from build123d import *

# Parameters (mm, degrees)
EXTRUDE_1_DEPTH     = 19
SKETCH_3_W          = 1
SKETCH_3_H          = 19
CUT_EXTRUDE_1_DEPTH = 1
SKETCH_4_R          = 2.25
CUT_EXTRUDE_2_DEPTH = 2
SKETCH_5_R          = 2.25
CUT_EXTRUDE_3_DEPTH = 2


with BuildPart() as part:
    # Эскиз1 → Бобышка-Вытянуть1 (new body)
    with BuildSketch(Plane(origin=(0, 0, 0), x_dir=(1, 0, 0), z_dir=(0, 1, 0))):
        Polygon((0, 0), (0, 20), (1, 20), (1, 1), (20, 1), (20, 0), align=None)
    extrude(amount=EXTRUDE_1_DEPTH)

    # Эскиз3 → Вырез-Вытянуть1 (cut)
    with BuildSketch(Plane(origin=(20, 0, 0), x_dir=(0, 0, -1), z_dir=(1, 0, 0))):
        with Locations((0.5, 9.5)):
            Rectangle(SKETCH_3_W, SKETCH_3_H)
    extrude(amount=-CUT_EXTRUDE_1_DEPTH, mode=Mode.SUBTRACT)

    # Эскиз4 → Вырез-Вытянуть2 (cut, through all)
    with BuildSketch(Plane(origin=(1, 0, 0), x_dir=(0, 0, -1), z_dir=(1, 0, 0))):
        with Locations((10.5, 9.5)):
            Circle(SKETCH_4_R)
    extrude(amount=-CUT_EXTRUDE_2_DEPTH, mode=Mode.SUBTRACT)

    # Эскиз5 → Вырез-Вытянуть3 (cut, through all)
    with BuildSketch(Plane(origin=(0, 0, -1), x_dir=(-1, 0, 0), z_dir=(0, 0, -1))):
        with Locations((-9, 9.5)):
            Circle(SKETCH_5_R)
    extrude(amount=-CUT_EXTRUDE_3_DEPTH, mode=Mode.SUBTRACT)


solid = part.part
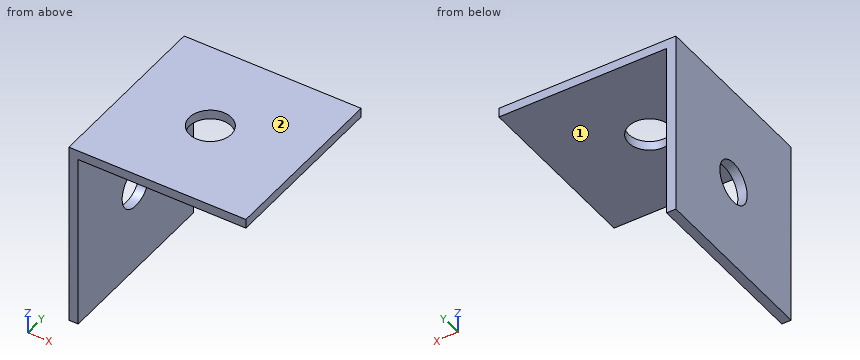
Source: CAD feature listing. Evaluate the final solid. Frame: model axes, mm. Face numbers are marked on the shaded views. A direction names the side the tool comes from. Round coordinates to 2 decimals unless told otherwise and drop trailing zeros. Write each loop counter-clockwise with the first axis right and the second up, starting at its lowest first coordinate (ties: lowest second). Pieces come first, ordered by that corner, then holes. Notation, with made-up numbers: M -9,-16.5 L 3,-16.5 A31 cw 3,18.5 Z; hole C -30.5,81.25 d11. An arc over 180 degrees is marked long. One line per item, written item: value. Start each with the question number.
Item 1: Section query A-A (y = 9.5). Return the cut outline in (x, z).
Item 2: Pin query (flat end, axial travel): pin 1 (1 mm diameter, centred on x = 16.5, y = 7, fed in from +Z); pin 2 (5 mm diameter, centred on y = 14, z = -11.5, fed in from +X); pin 3 (1 mm diameter, centred on x = 9.5, y = 16, fed in from -Z). Return the tip coordinate at first contact, or that it passes through.
Item 3: Section query D-D (x = 17.5). Return the cut outline in (y, z), plus the area to 3 significant figures.
Item 4: Ray query, L1, parallel to Y at x = 0.75, z = -10.5; L2, parallel to X at y = 12.75, z = -16; L3, parallel to Z at x = 14.25, y = 5.25. Return the intervals inside material, ascending. Write a range as from..to.
Item 5: Set-up query: the marked faces 1 and 2. Return all of +Z, -Z, +X, -X, +Y, -Y with unobstructed straight access to the full face (end or side cutting, diameter ignored); none if empty.
Item 6: Section query C-C (z = -10.5). Return the cut outline in (x, y).
Item 7: Section query B-B (x = 9). Return the cut outline in (y, z), plus the area to 3 significant figures.
Result set:
1. outline: M 0,-20 L 1,-20 L 1,-12.75 L 0,-12.75 Z; M 0,-8.25 L 1,-8.25 L 1,-1 L 6.75,-1 L 6.75,0 L 0,0 Z; M 11.25,-1 L 19,-1 L 19,0 L 11.25,0 Z
2. pin 1: stops at z = 0
2. pin 2: stops at x = 1
2. pin 3: stops at z = -1
3. outline: M 0,-1 L 19,-1 L 19,0 L 0,0 Z
3. area: 19.0 mm²
4. L1: y = 0..7.25, 11.75..19
4. L2: x = 0..1
4. L3: z = -1..0
5. face 1: -Z, +X, +Y, -Y
5. face 2: +Z, +X, -X, +Y, -Y
6. outline: M 0,0 L 1,0 L 1,7.25 L 0,7.25 Z; M 0,11.75 L 1,11.75 L 1,19 L 0,19 Z
7. outline: M 0,-1 L 7.25,-1 L 7.25,0 L 0,0 Z; M 11.75,-1 L 19,-1 L 19,0 L 11.75,0 Z
7. area: 14.5 mm²
